Autodesk Inventor part; units mm, degrees
ref_plane "YZ Plane" through (0, 0, 0) normal (1, 0, 0) x (0, 1, 0)
ref_plane "XZ Plane" through (0, 0, 0) normal (0, 1, 0) x (-1, 0, 0)
ref_plane "XY Plane" through (0, 0, 0) normal (0, 0, 1) x (1, 0, 0)
sketch "Sketch1" plane through (0, 0, 0) normal (0, 1, 0) x (-1, 0, 0)
  line L0 (-95, 95) -> (95, 95)
  line L1 (95, 95) -> (95, -95)
  line L2 (95, -95) -> (-95, -95)
  line L3 (-95, -95) -> (-95, 95)
  line L4 (-95, 95) -> (95, -95) construction
  line L5 (95, 95) -> (-95, -95) construction
  point P0 (0, 0)
  dimension "d0" = 190
  dimension "d1" = 190
extrude "Extrusion1" add sketch "Sketch1" along normal blind 5
sketch "Sketch2" plane through (0, 5, 0) normal (0, 1, 0) x (1, 0, 0)
  line L0 (-15, -15) -> (15, -15)
  line L1 (15, -15) -> (15, 15)
  line L2 (15, 15) -> (-15, 15)
  line L3 (-15, 15) -> (-15, -15)
  line L4 (-15, -15) -> (15, 15) construction
  line L5 (15, -15) -> (-15, 15) construction
  point P0 (0, 0)
  dimension "d4" = 30
  dimension "d5" = 30
extrude "Extrusion2" add sketch "Sketch2" along normal blind 12
sketch "Sketch3" plane through (0, 17, 0) normal (0, 1, 0) x (1, 0, 0)
  line L0 (-10, -2.5) -> (-4.3301, -2.5)
  line L1 (10, -2.5) -> (10, 2.5)
  line L2 (10, 2.5) -> (4.3301, 2.5)
  line L3 (-10, 2.5) -> (-10, -2.5)
  line L4 (-10, -2.5) -> (10, 2.5) construction
  line L5 (10, -2.5) -> (-10, 2.5) construction
  arc A0 (-4.3301, -2.5) -> (4.3301, -2.5) centre (0, 0) ccw
  arc A1 (4.3301, 2.5) -> (-4.3301, 2.5) centre (0, 0) ccw
  line L6 (4.3301, -2.5) -> (10, -2.5)
  line L7 (-4.3301, 2.5) -> (-10, 2.5)
  dimension "d9" = 20
  dimension "d10" = 5
extrude "Extrusion3" cut sketch "Sketch3" against normal blind 11
fillet "Fillet1" radius 5 4 edges at (-95, 2.5, 95) (-95, 2.5, -95) (95, 2.5, 95) (95, 2.5, -95)
fillet "Fillet2" radius 5 4 edges at (-15, 11, 15) (15, 11, 15) (15, 11, -15) (-15, 11, -15)
sketch "Sketch5" plane through (0, 5, 0) normal (0, 1, 0) x (1, 0, 0)
  line L0 (-15, -10) -> (-15, 10)
  arc A0 (-10, 15) -> (-15, 10) centre (-10, 10) ccw
  line L1 (-10, 15) -> (10, 15)
  arc A1 (15, 10) -> (10, 15) centre (10, 10) ccw
  line L2 (15, 10) -> (15, -10)
  arc A2 (10, -15) -> (15, -10) centre (10, -10) ccw
  line L3 (10, -15) -> (-10, -15)
  arc A3 (-15, -10) -> (-10, -15) centre (-10, -10) ccw
  arc A4 (95, 90) -> (90, 95) centre (90, 90) ccw
  line L4 (90, 95) -> (-90, 95)
  arc A5 (-90, 95) -> (-95, 90) centre (-90, 90) ccw
  line L5 (-95, 90) -> (-95, -90)
  arc A6 (-95, -90) -> (-90, -95) centre (-90, -90) ccw
  line L6 (-90, -95) -> (90, -95)
  arc A7 (90, -95) -> (95, -90) centre (90, -90) ccw
  line L7 (95, -90) -> (95, 90)
  arc A8 (15, 10) -> (10, 15) centre (10, 10) ccw
  line L8 (38.9645, 46.0355) -> (17.9289, 25)
  line L9 (38.9645, 46.0355) -> (77.9289, 85)
  line L10 (-38.9645, 46.0355) -> (-17.9289, 25)
  line L11 (-38.9645, 46.0355) -> (-77.9289, 85)
  line L12 (-77.9289, 85) -> (77.9289, 85)
  line L13 (17.9289, 25) -> (-17.9289, 25)
  line L14 (-4.3301, -2.5) -> (-10, -2.5)
  arc A9 (-4.3301, -2.5) -> (4.3301, -2.5) centre (0, 0) ccw
  line L15 (10, -2.5) -> (4.3301, -2.5)
  line L16 (10, 2.5) -> (10, -2.5)
  line L17 (4.3301, 2.5) -> (10, 2.5)
  arc A10 (4.3301, 2.5) -> (-4.3301, 2.5) centre (0, 0) ccw
  line L18 (-10, 2.5) -> (-4.3301, 2.5)
  line L19 (-10, -2.5) -> (-10, 2.5)
  line L20 (-4.3301, -2.5) -> (-10, -2.5)
  arc A11 (-4.3301, -2.5) -> (4.3301, -2.5) centre (0, 0) ccw
  line L21 (10, -2.5) -> (4.3301, -2.5)
  line L22 (10, 2.5) -> (10, -2.5)
  line L23 (4.3301, 2.5) -> (10, 2.5)
  arc A12 (4.3301, 2.5) -> (-4.3301, 2.5) centre (0, 0) ccw
  line L24 (-10, 2.5) -> (-4.3301, 2.5)
  line L25 (-10, -2.5) -> (-10, 2.5)
  arc A13 (4.3301, 2.5) -> (-4.3301, 2.5) centre (0, 0) ccw
  arc A14 (-4.3301, -2.5) -> (4.3301, -2.5) centre (0, 0) ccw
  line L26 (25, -17.9289) -> (25, 17.9289)
  line L27 (85, 77.9289) -> (85, -77.9289)
  line L28 (46.0355, -38.9645) -> (25, -17.9289)
  line L29 (46.0355, -38.9645) -> (85, -77.9289)
  line L30 (46.0355, 38.9645) -> (85, 77.9289)
  line L31 (46.0355, 38.9645) -> (25, 17.9289)
  line L32 (-17.9289, -25) -> (17.9289, -25)
  line L33 (77.9289, -85) -> (-77.9289, -85)
  line L34 (-38.9645, -46.0355) -> (-17.9289, -25)
  line L35 (-38.9645, -46.0355) -> (-77.9289, -85)
  line L36 (38.9645, -46.0355) -> (77.9289, -85)
  line L37 (38.9645, -46.0355) -> (17.9289, -25)
  line L38 (-25, 17.9289) -> (-25, -17.9289)
  line L39 (-85, -77.9289) -> (-85, 77.9289)
  line L40 (-46.0355, 38.9645) -> (-25, 17.9289)
  line L41 (-46.0355, 38.9645) -> (-85, 77.9289)
  line L42 (-46.0355, -38.9645) -> (-85, -77.9289)
  line L43 (-46.0355, -38.9645) -> (-25, -17.9289)
  dimension "d24" = 360
extrude "Extrusion4" cut sketch "Sketch5" against normal blind 32.75 contours L8 L13 L10 L11 L12 L9 | L26 L31 L30 L27 L29 L28 | L32 L37 L36 L33 L35 L34 | L38 L43 L42 L39 L41 L40
fillet "Fillet3" radius 5 16 edges at (85, 2.5, -77.9289) (77.9289, 2.5, -85) (-85, 2.5, -77.9289) (-77.9289, 2.5, -85) (-17.9289, 2.5, -25) (17.9289, 2.5, -25) (-25, 2.5, -17.9289) (-17.9289, 2.5, 25) (17.9289, 2.5, 25) (85, 2.5, 77.9289) (77.9289, 2.5, 85) (-77.9289, 2.5, 85) (-85, 2.5, 77.9289) (-25, 2.5, 17.9289) (25, 2.5, 17.9289) (25, 2.5, -17.9289)
properties part number "Base"
Can you work these out from the model? Positions are in its coordinate system, mm. A direction names the side the tool comes from. Give positions to 0.01 mm unless a question says otherwise; leave off trailing zeros. Order: outer loops, then holes, each group sorted by start corner. A loop starts at its lowest first (then second) coordinate and runs counter-clockwise, first axis right, second up. Notation, with made-up numbers: (5, 12) - (45, 12) arc R14 ccw to (45, 33) - close; hole circle Ø9 at (0.5, 52). An arc over 180 degrees is marked (long way). Use a Markdown table: item, result. Add a question column.
Q1. If we section it at D-D on x = 74: Write out the boundary of the cut face in (y, z).
Q2. If we section it at A-A on y = 10.75: Write out the boundary of the cut face in (x, z), plus the area to 3 significant figures.
Q3. I'm going to push flat-ended pins straight in: pin 1 (3.5 mm diameter, centred on x = -0.5, y = 11, fed in from -Z); pin 2 (1.5 mm diameter, centred on y = 13, z = -1, fed in from +X); pin 3 (1 mm diameter, centred on x = -7.5, y = 14, fed in from +Z). Where does each tip first touch, or does it pass through?
Q4. If we section it at B-B on x = -1.5: Write out the boundary of the cut face in (y, z), plus the area to 3 significant figures.
Q5. On a 3-axis mill with a long thin cutter (end or side, diameter ignored), from which of +Z, -Z, +X, -X, +Y, -Y can I reach the whole of each face in a straight line? I mean faces 5 (the cylindrical face through (0, 12, -5)), 6 (the flat face through (0, 3, -25)), 7 (the flat face through (0, 11, 15)), 8 (the cylindrical face through (13, 11, 14)). Say none if no direction works.
Q6. Please list where these lines run through material, in increasing order: line 1 along X through (y, z) = (4.75, 30); line 2 along Z through (x, y) = (-35.5, 4); line 3 along Z through (x, y) = (53, 3.5).
Q7. If we mould it in two halves opening along X, with no side actions, what happens to faces 1 (the cylindrical face through (-93, 3, -94)), 2 (the cylindrical face through (14, 11, -13)), 3 (the flat face through (1, 2, 95)), 4 (the cylindrical face through (-70.508, 2.465, -81.837))? For each: released by +X, released by -X, zero draft, split by the parting line, or undercut.
Q8. If we section it at C-C on z = -59.5: Write out the boundary of the cut face in (x, y), plus the area to 3 significant figures.
Answers follow:
| question | item | result |
|---|---|---|
| 1 | outline | (0, -95) - (5, -95) - (5, -66.93) - (0, -66.93) - close; (0, 66.93) - (5, 66.93) - (5, 95) - (0, 95) - close |
| 2 | outline | (-15, -10) arc R5 ccw to (-10, -15) - (10, -15) arc R5 ccw to (15, -10) - (15, 10) arc R5 ccw to (10, 15) - (-10, 15) arc R5 ccw to (-15, 10) - close; hole (-10, -2.5) - (-4.33, -2.5) arc R5 ccw to (4.33, -2.5) - (10, -2.5) - (10, 2.5) - (4.33, 2.5) arc R5 ccw to (-4.33, 2.5) - (-10, 2.5) - close |
| 2 | area | 748 mm^2 |
| 3 | pin 1 | stops at z = -15 |
| 3 | pin 2 | stops at x = 15 |
| 3 | pin 3 | stops at z = 15 |
| 4 | outline | (0, -95) - (5, -95) - (5, -85) - (0, -85) - close; (0, -25) - (5, -25) - (5, -15) - (17, -15) - (17, -4.77) - (6, -4.77) - (6, 4.77) - (17, 4.77) - (17, 15) - (5, 15) - (5, 25) - (0, 25) - close; (0, 85) - (5, 85) - (5, 95) - (0, 95) - close |
| 4 | area | 605 mm^2 |
| 5 | face 5 | +Y |
| 5 | face 6 | +Y, -Y |
| 5 | face 7 | +Z, +X, -X, +Y |
| 5 | face 8 | +Z, +X, +Y |
| 6 | line 1 | x = -95 to -85, -37.07 to -22.93, 22.93 to 37.07, 85 to 95 |
| 6 | line 2 | z = -95 to -85, -42.57 to -28.43, 28.43 to 42.57, 85 to 95 |
| 6 | line 3 | z = -95 to -85, -60.07 to -45.93, 45.93 to 60.07, 85 to 95 |
| 7 | face 1 | released by -X |
| 7 | face 2 | released by +X |
| 7 | face 3 | zero draft |
| 7 | face 4 | undercut |
| 8 | outline | (-95, 0) - (-85, 0) - (-85, 5) - (-95, 5) - close; (-66.57, 0) - (-52.43, 0) - (-52.43, 5) - (-66.57, 5) - close; (52.43, 0) - (66.57, 0) - (66.57, 5) - (52.43, 5) - close; (85, 0) - (95, 0) - (95, 5) - (85, 5) - close |
| 8 | area | 241 mm^2 |
